from build123d import *

# Parameters (mm, degrees)
F1_DEPTH    = 110
F2_T1_DEPTH = 380.0356183152


# Not quite as in the source:
# - a fillet or chamfer that OpenCascade refuses, or shapes differently, is made with other operations: its cross-section is extruded or revolved along the edge and cut away or added


with BuildPart() as f1:
    # F0 (on Right) → F1 (new body)
    with BuildSketch(Plane.YZ):
        Polygon((-60, 0), (0, 0), (0, 60), (-20, 60), (-20, 40), (-40, 40), (-40, 20), (-60, 20), align=None)
    extrude(amount=F1_DEPTH)

    # F2: chamfer of 70 on 1 edges, made by hand

    # F2_s2 → F2_t1 (cut)
    with BuildSketch(Plane.XZ.offset(-180.0178091576)):
        Polygon((40, 60), (110, -10), (110, 60), align=None)
    extrude(amount=F2_T1_DEPTH, mode=Mode.SUBTRACT)


solid = f1.part
Geometry: final body of the model. Coordinates: model frame, mm. A direction names the side the tool comes from. Round coordinates to 2 decimals unless told otherwise and drop trailing zeros. Order: outer loops, then holes, each group sorted by start corner. A loop starts at its lowest first (then second) coordinate and runs counter-clockwise, first axis right, second up.
Q1. Material intervals for probe 1 along Z at (x, y) = (57.5, -51); probe 2 along Z at (x, y) = (36, -21); probe 3 along Y at (x, z) = (34, 25), sorted ascending.
Result sheet:
probe 1: z = 0 to 20
probe 2: z = 0 to 40
probe 3: y = -40 to 0
Q2. Section D-D, the plane x = 41.5. Output: boundary loops of the cut face in (y, z).
Result sheet:
outline: (-60, 0) - (0, 0) - (0, 58.5) - (-20, 58.5) - (-20, 40) - (-40, 40) - (-40, 20) - (-60, 20) - close
Q3. Section B-B, the plane y = -14. Output: boundary loops of the cut face in (x, z).
Result sheet:
outline: (0, 0) - (100, 0) - (40, 60) - (0, 60) - close
Q4. Access query for faces 1 (the face through (23, -20, 50)), 2 (the face through (20, -10, 60)). Directions: +Z, -Z, +X, -X, +Y, -Y. A direction counts if a zero-diameter tool reaches every point of the face in a straight line with its end or side. Return the directions, or none.
Result sheet:
face 1: +Z, +X, -X, -Y
face 2: +Z, +X, -X, +Y, -Y
Q5. Section C-C, the plane z = 55. Output: boundary loops of the cut face in (x, y).
Result sheet:
outline: (0, -20) - (45, -20) - (45, 0) - (0, 0) - close
Q6. Section A-A, the plane x = 14. Output: boundary loops of the cut face in (y, z).
Result sheet:
outline: (-60, 0) - (0, 0) - (0, 60) - (-20, 60) - (-20, 40) - (-40, 40) - (-40, 20) - (-60, 20) - close
Q7. Pin query (flat end, axial travel): pin 1 (1.5 mm diameter, centred on x = 41, z = 22, fed in from -Y); pin 2 (3 mm diameter, centred on y = -10, z = 33.5, fed in from -X); pin 3 (12 mm diameter, centred on y = -17, z = 28.5, fed in from +X); pin 4 (6 mm diameter, centred on x = 34.5, y = -28, fed in from +Z). Return the tip coordinate at first contact, or that it passes through.
Result sheet:
pin 1: stops at y = -40
pin 2: stops at x = 0
pin 3: stops at x = 77.5
pin 4: stops at z = 40
